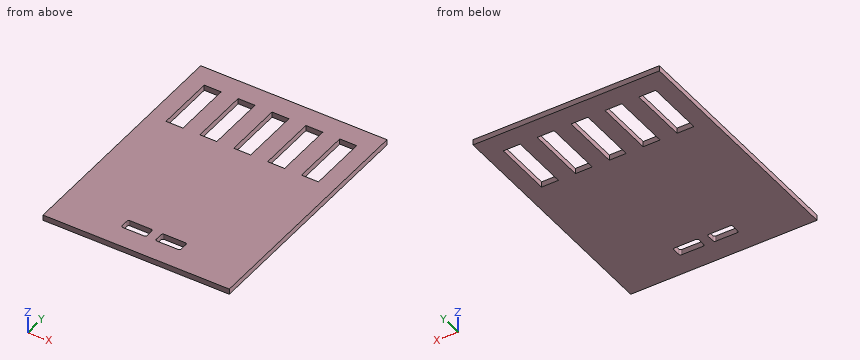
```python
from build123d import *

# Parameters (mm, degrees)
SKETCH1_W           = 101
SKETCH1_H           = 132
BOSS_EXTRUDE1_DEPTH = 1.5
SKETCH2_W           = 9.181818182
SKETCH2_H           = 32
CUT_EXTRUDE1_DEPTH  = 84.157982179


with BuildPart() as part:
    # Sketch1 → Boss-Extrude1 (new, symmetric)
    with BuildSketch(Plane.XY):
        Rectangle(SKETCH1_W, SKETCH1_H)
    extrude(amount=BOSS_EXTRUDE1_DEPTH, both=True)

    # Sketch2 → Cut-Extrude1 (cut, through all)
    with BuildSketch(Plane.XY.offset(1.5)):
        with BuildLine():
            Line((3.5, -54), (15, -54))
            ThreePointArc((15, -54), (15.707106781, -53.707106781), (16, -53))
            Line((16, -53), (16, -49))
            ThreePointArc((16, -49), (15.707106781, -48.292893219), (15, -48))
            Line((15, -48), (3.5, -48))
            ThreePointArc((3.5, -48), (2.792893219, -48.292893219), (2.5, -49))
            Line((2.5, -49), (2.5, -53))
            ThreePointArc((2.5, -53), (2.792893219, -53.707106781), (3.5, -54))
        make_face()
        with Locations((-36.727272727, 38.8)):
            Rectangle(SKETCH2_W, SKETCH2_H)
        with Locations((-18.363636364, 38.8)):
            Rectangle(SKETCH2_W, SKETCH2_H)
        with Locations((0, 38.8)):
            Rectangle(SKETCH2_W, SKETCH2_H)
        with Locations((18.363636364, 38.8)):
            Rectangle(SKETCH2_W, SKETCH2_H)
        with Locations((36.727272727, 38.8)):
            Rectangle(SKETCH2_W, SKETCH2_H)
        with BuildLine():
            Line((-15, -54), (-3.5, -54))
            ThreePointArc((-3.5, -54), (-2.792893219, -53.707106781), (-2.5, -53))
            Line((-2.5, -53), (-2.5, -49))
            ThreePointArc((-2.5, -49), (-2.792893219, -48.292893219), (-3.5, -48))
            Line((-3.5, -48), (-15, -48))
            ThreePointArc((-15, -48), (-15.707106781, -48.292893219), (-16, -49))
            Line((-16, -49), (-16, -53))
            ThreePointArc((-16, -53), (-15.707106781, -53.707106781), (-15, -54))
        make_face()
    extrude(amount=-CUT_EXTRUDE1_DEPTH, mode=Mode.SUBTRACT)


solid = part.part
```
Geometry check sheet. Reference: the model listing, model coordinates, mm. Coordinates: 2 decimals unless noted, no trailing zeros. Loops run counter-clockwise (first coordinate to the right, second up) from the corner with the lowest first, then second, coordinate; pieces in that order, holes last. Notation, with made-up numbers: (88.25, 62.5) -> (147.25, 62.5) arc R9 ccw to (147.25, 75.5) -> close; hole circle Ø4 at (68.5, -11.75). An arc over 180 degrees is marked (long way). Put each result on its own line as item: value.
1) Cross-section at C-C on z = 0.9. Count the separate pieces of the cut face and the enclosed holes in it, plus the area to 3 significant figures.
Result set:
separate pieces: 1
enclosed holes: 7
area: 11,700 mm^2
2) Cross-section at B-B on y = 28. Record the boundary of the cut face in (x, z), plus the area to 3 significant figures.
Result set:
outline: (-50.5, -1.5) -> (-41.32, -1.5) -> (-41.32, 1.5) -> (-50.5, 1.5) -> close; (-32.14, -1.5) -> (-22.95, -1.5) -> (-22.95, 1.5) -> (-32.14, 1.5) -> close; (-13.77, -1.5) -> (-4.59, -1.5) -> (-4.59, 1.5) -> (-13.77, 1.5) -> close; (4.59, -1.5) -> (13.77, -1.5) -> (13.77, 1.5) -> (4.59, 1.5) -> close; (22.95, -1.5) -> (32.14, -1.5) -> (32.14, 1.5) -> (22.95, 1.5) -> close; (41.32, -1.5) -> (50.5, -1.5) -> (50.5, 1.5) -> (41.32, 1.5) -> close
area: 165 mm^2
3) Cross-section at A-A on x = -1. Record the boundary of the cut face in (y, z).
Result set:
outline: (-66, -1.5) -> (22.8, -1.5) -> (22.8, 1.5) -> (-66, 1.5) -> close; (54.8, -1.5) -> (66, -1.5) -> (66, 1.5) -> (54.8, 1.5) -> close
4) Thickness scan on line 1 (X direction, y = 24.5, z = 1.3); line 2 (X direction, y = -51.5, z = 0.55); line 3 (Y direction, x = 21, z = -0.15). Record the ranges inside material, lowest first.
Result set:
line 1: x = -50.5 to -41.32, -32.14 to -22.95, -13.77 to -4.59, 4.59 to 13.77, 22.95 to 32.14, 41.32 to 50.5
line 2: x = -50.5 to -16, -2.5 to 2.5, 16 to 50.5
line 3: y = -66 to 22.8, 54.8 to 66
